Model file for the job. Use its own axes, mm. Face numbers are marked on the shaded views. A direction names the side the tool comes from. Give positions to 0.01 mm unless a question says otherwise; leave off trailing zeros. Order: outer loops, then holes, each group sorted by start corner. A loop starts at its lowest first (then second) coordinate and runs counter-clockwise, first axis right, second up. Notation, with made-up numbers: (-12, 66) - (-5, 66) arc R22 cw to (-5, 98) - close; hole circle Ø3 at (18, -28.75). An arc over 180 degrees is marked (long way). Use CSV: the item, a comma, the result in double quotes. Start each with the question number.
(1) Probe L1, parallel to Y at x = -35.75, z = 12.25; L2, parallel to Y at x = -0.5, z = 16.5; L3, parallel to X at y = -1, z = 2.5. List the from-to ranges inside material, lowest first.
(2) Band-saw the part on C-C, the plane y = 25. Give the cut face in (x, z).
(3) Tool access for the marked faces 1, 2, 3, 4 and 5: list every direction of +Z, -Z, +X, -X, +Y, -Y with a clear straight run to the whole face (end or side of a thin tool).
(4) Band-saw the part on A-A, the plane z = 5.5. Count the separate pieces of the cut face and the enclosed holes in it, then the cut area to 3 significant figures.
(5) Drop flat-ended pins along their axis: pin 1 Ø7.5 at (y, z) = (25, 5) entering from -X; pin 2 Ø8 at (y, z) = (20, 8) entering from +X; pin 3 Ø7.5 at (y, z) = (-23.5, 12) entering from +X; pin 4 Ø2.5 at (x, y) = (35.75, 35.75) entering from +Z. Give the stop position or say it passes through.
(6) Band-saw the part on B-B, the plane x = -36. Give the cut face in (y, z).
(7) Band-saw the part on D-D, the plane x = -7. Give the cut face in (y, z), then the cut area to 3 significant figures.
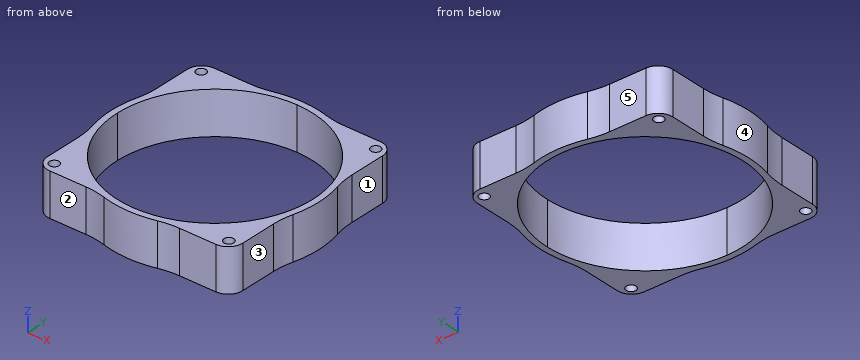
from build123d import *

# Parameters (mm, degrees)
F0_R     = 2
F1_DEPTH = 17.5
F2_R     = 6
F3_R     = 32


with BuildPart() as f1:
    # F0 (on Top) → F1 (new body)
    with BuildSketch(Plane.XY):
        with BuildLine():
            Line((40, 14.3614066163), (40, 40))
            Line((40, 40), (14.3614066163, 40))
            ThreePointArc((14.3614066163, 40), (30.0520382004, 30.0520382004), (40, 14.3614066163))
        make_face()
        with Locations((35.75, 35.75)):
            Circle(F0_R, mode=Mode.SUBTRACT)
        with BuildLine():
            ThreePointArc((40, 14.3614066163), (30.0520382004, 30.0520382004), (14.3614066163, 40))
            Line((14.3614066163, 40), (0, 40))
            ThreePointArc((0, 40), (28.2842712475, 28.2842712475), (40, 0))
            Line((40, 0), (40, 14.3614066163))
        make_face()
        with BuildLine():
            Line((0, 40), (14.3614066163, 40))
            ThreePointArc((14.3614066163, 40), (0, 42.5), (-14.3614066163, 40))
            Line((-14.3614066163, 40), (0, 40))
        make_face()
        with BuildLine():
            ThreePointArc((42.5, 0), (41.8703355611, 7.2886898686), (40, 14.3614066163))
            Line((40, 14.3614066163), (40, 0))
            Line((40, 0), (40, -14.3614066163))
            ThreePointArc((40, -14.3614066163), (41.8703355611, -7.2886898686), (42.5, 0))
        make_face()
        with BuildLine():
            ThreePointArc((-40, 0), (-28.2842712475, 28.2842712475), (0, 40))
            Line((0, 40), (-14.3614066163, 40))
            ThreePointArc((-14.3614066163, 40), (-30.0520382004, 30.0520382004), (-40, 14.3614066163))
            Line((-40, 14.3614066163), (-40, 0))
        make_face()
        with BuildLine():
            ThreePointArc((-40, 14.3614066163), (-30.0520382004, 30.0520382004), (-14.3614066163, 40))
            Line((-14.3614066163, 40), (-40, 40))
            Line((-40, 40), (-40, 14.3614066163))
        make_face()
        with Locations((-35.75, 35.75)):
            Circle(F0_R, mode=Mode.SUBTRACT)
        with BuildLine():
            Line((40, -14.3614066163), (40, 0))
            ThreePointArc((40, 0), (28.2842712475, -28.2842712475), (0, -40))
            Line((0, -40), (14.3614066163, -40))
            ThreePointArc((14.3614066163, -40), (30.0520382004, -30.0520382004), (40, -14.3614066163))
        make_face()
        with BuildLine():
            Line((-40, -14.3614066163), (-40, 0))
            Line((-40, 0), (-40, 14.3614066163))
            ThreePointArc((-40, 14.3614066163), (-42.5, 0), (-40, -14.3614066163))
        make_face()
        with BuildLine():
            ThreePointArc((0, -40), (-28.2842712475, -28.2842712475), (-40, 0))
            Line((-40, 0), (-40, -14.3614066163))
            ThreePointArc((-40, -14.3614066163), (-30.0520382004, -30.0520382004), (-14.3614066163, -40))
            Line((-14.3614066163, -40), (0, -40))
        make_face()
        with BuildLine():
            Line((40, -40), (40, -14.3614066163))
            ThreePointArc((40, -14.3614066163), (30.0520382004, -30.0520382004), (14.3614066163, -40))
            Line((14.3614066163, -40), (40, -40))
        make_face()
        with Locations((35.75, -35.75)):
            Circle(F0_R, mode=Mode.SUBTRACT)
        with BuildLine():
            Line((14.3614066163, -40), (0, -40))
            Line((0, -40), (-14.3614066163, -40))
            ThreePointArc((-14.3614066163, -40), (0, -42.5), (14.3614066163, -40))
        make_face()
        with BuildLine():
            ThreePointArc((-14.3614066163, -40), (-30.0520382004, -30.0520382004), (-40, -14.3614066163))
            Line((-40, -14.3614066163), (-40, -40))
            Line((-40, -40), (-14.3614066163, -40))
        make_face()
        with Locations((-35.75, -35.75)):
            Circle(F0_R, mode=Mode.SUBTRACT)
    extrude(amount=F1_DEPTH)

    # F2
    f2_edges = [f1.edges().sort_by_distance(p)[0] for p in [
        (-40, -40, 8.75),
        (40, -40, 8.75),
        (-40, 40, 8.75),
        (40, 40, 8.75),
    ]]
    fillet(f2_edges, radius=F2_R)

    # F3
    f3_edges = [f1.edges().sort_by_distance(p)[0] for p in [
        (-40, 14.361407, 8.75),
        (-40, -14.361407, 8.75),
        (-14.361407, -40, 8.75),
        (14.361407, -40, 8.75),
        (40, -14.361407, 8.75),
        (40, 14.361407, 8.75),
        (14.361407, 40, 8.75),
        (-14.361407, 40, 8.75),
    ]]
    fillet(f3_edges, radius=F3_R)


solid = f1.part
Answer block:
1,L1,"y = -39.74 to -37.75, -33.75 to -17.94, 17.94 to 33.75, 37.75 to 39.74"
1,L2,"y = -42.5 to -40, 40 to 42.5"
1,L3,"x = -42.49 to -39.99, 39.99 to 42.49"
2,outline,"(-40, 0) - (-31.22, 0) - (-31.22, 17.5) - (-40, 17.5) - close; (31.22, 0) - (40, 0) - (40, 17.5) - (31.22, 17.5) - close"
3,face 1,"+Z, -Z, +X, +Y"
3,face 2,"+Z, -Z, -X, -Y"
3,face 3,"+Z, -Z, +X, -Y"
3,face 4,"+Z, -Z, -X"
3,face 5,"+Z, -Z, -X, +Y"
4,separate pieces,"1"
4,enclosed holes,"5"
4,area,"1,490 mm2"
5,pin 1,"stops at x = -40"
5,pin 2,"stops at x = 40.15"
5,pin 3,"stops at x = 40"
5,pin 4,"passes through"
6,outline,"(-39.66, 0) - (-37.73, 0) - (-37.73, 17.5) - (-39.66, 17.5) - close; (-33.77, 0) - (-17.44, 0) - (-17.44, 17.5) - (-33.77, 17.5) - close; (17.44, 0) - (33.77, 0) - (33.77, 17.5) - (17.44, 17.5) - close; (37.73, 0) - (39.66, 0) - (39.66, 17.5) - (37.73, 17.5) - close"
7,outline,"(-41.92, 0) - (-39.38, 0) - (-39.38, 17.5) - (-41.92, 17.5) - close; (39.38, 0) - (41.92, 0) - (41.92, 17.5) - (39.38, 17.5) - close"
7,area,"88.8 mm2"
